For this review, take the finished solid that the model builds, in its own axes (mm). A direction names the side the tool comes from. Give positions to 0.01 mm unless a question says otherwise; leave off trailing zeros. Order: outer loops, then holes, each group sorted by start corner. A loop starts at its lowest first (then second) coordinate and runs counter-clockwise, first axis right, second up. Notation, with made-up numbers: (25, -34) - (56, -34) arc R20 cw to (56, -12) - close; hole circle Ø1 at (34, 16.25). An arc over 180 degrees is marked (long way). Use a Markdown table: item, result. Add a question column.
1) We need section A-A on x = 4.75. Write out the cut boundary in (y, z).
2) Machinability: for faces 4 (the face through (-7.25, 0.65, 0.5)), 5 (the face through (-1, 7, 0)), 6 (the face through (-4.61, -4.987, 0.501)), 7 (the face through (-6.28, 4.25, 0.5)), which of the approach directions +Z, -Z, +X, -X, +Y, -Y give a long, thin tool a straight path to every point of the face, cutting with its end or side? Answer none if there is none.
3) Wall thickness on L1, parallel to Z at x = 2.25, y = -4.25; L2, parallel to Z at x = 5, y = -6.5; L3, parallel to Y at x = 6.75, z = 0.4: over which ranges is each line inside the solid? List them lowest first.
4) We need section B-B on z = -1. Write out the cut boundary in (x, y) (3 decimals), then the cut area to 3 significant figures.
5) Clearance check with flat-ended pins moving along their axes: P1, Ø1, axis at y = 4.5, z = -1.5, coming from the -X side; P2, Ø0.5, axis at x = 0, z = 0.5, coming from the -Y side; P3, Ø7, axis at x = -0.5, y = -3.5, coming from the +Z side; P4, Ø0.5, axis at y = 0.5, z = 0.5, coming from the +X side. State where each tip first meets the part, or that it passes through.
6) Mouldability with a two-part tool opening along X and no side actions: class faces 1 (the face through (-0.1, -8.666, 0.5)), 2 (the face through (-2.85, -7.1, 0.5)), 3 (the face through (0, 1, 0.762)) as released by +X, released by -X, zero draft, split by the parting line, or undercut.
```python
from build123d import *

# Parameters (mm, degrees)
F2_DEPTH  = 1.016
F0_R      = 9.525
F3_DEPTH  = 1.778
F5_DEPTH  = 0.73658
F8_DEPTH  = 0.19799
F10_DEPTH = 0.254
F12_DEPTH = 0.254
F14_DEPTH = 0.254
F16_DEPTH = 0.13808
F18_DEPTH = 0.254


with BuildPart() as f2:
    # F1 (on Top) → F2 (new body)
    with BuildSketch(Plane.XY):
        Polygon((-5.2096517757, 4.8718452454), (-7.3895002715, 3.6098279525), (-6.5481550992, 2.3594415264), (-6.86526423, 2.3594415264), (-7.3371550568, 1.5301066978), (-6.8923411891, 1.2770079775), (-7.6189576648, 0), (-7.6189576648, -0.3674388281), (-7.1600424126, -2.2795863915), (-6.7776124924, -3.1974171288), (-5.4391096346, -4.4211917557), (-3.7564195227, -5.5684801191), (-1.9207580481, -8.6661595851), (1.8270511646, -8.6661595851), (4.0068994276, -5.4537514225), (5.4983743466, -4.6506496146), (7.0280926302, -2.9297166038), (7.639979478, -1.7441851087), (7.639979478, -0.7116254419), (7.639979478, 0.3974201391), (7.639979478, 1.0475503514), (7.639979478, 1.6976804473), (6.4162053168, 2.4625393562), (7.6782228425, 3.6098279525), (5.6895888411, 4.5659020543), (4.427571781, 5.7131904177), (3.471497912, 6.1338627711), (1.6740793362, 7.0134503767), (0, 6.36332063), (-1.5000854619, 6.9752074778), (-3.2975040376, 6.17210567), (-4.3683070689, 5.5219754577), align=None)
    extrude(amount=F2_DEPTH)

    # F0 (on Top) → F3 (join)
    with BuildSketch(Plane.XY):
        Circle(F0_R)
    extrude(amount=-F3_DEPTH)

    # F7 (on face) → F8 (cut)
    with BuildSketch(Plane.XY.offset(1.016)):
        Polygon((-1.3463342329, 6.4942925237), (-2.822693903, 5.8646216057), (-2.6447118726, 5.755500868), (-1.3636830263, 6.2029086985), (0, 5.3883814253), (1.3446520315, 6.2008285895), (2.729951404, 5.569380708), (2.881785389, 5.6656086817), (1.3232411584, 6.5193735063), (0, 5.8390707709), align=None)
    extrude(amount=-F8_DEPTH, mode=Mode.SUBTRACT)

    # F9 (on face) → F10 (cut)
    with BuildSketch(Plane.XY.offset(1.016)):
        Polygon((-3.0135090929, -4.5730909333), (-2.8008187655, -4.5092836954), (-3.4176206682, -2.6801475324), (-4.5236102305, -2.1271528676), (-5.7784831151, -0.2554782841), (-5.1404121332, 0.4251306527), (-5.4594473913, 1.2333536288), (-5.246757064, 2.679647645), (-5.5232541636, 2.679647645), (-6.3314777799, 0.5314758164), (-6.3314777799, -1.0211633053), (-4.0769609623, -3.9137513377), (-3.545235144, -3.9137513377), align=None)
        Polygon((5.5232541636, 2.679647645), (5.246757064, 2.679647645), (5.4594473913, 1.2333536288), (5.1404121332, 0.4251306527), (5.7784831151, -0.2554782841), (4.5236102305, -2.1271528676), (3.4176206682, -2.6801475324), (2.8008187655, -4.5092836954), (3.0135090929, -4.5730909333), (3.545235144, -3.9137513377), (4.0769609623, -3.9137513377), (6.3314777799, -1.0211633053), (6.3314777799, 0.5314758164), align=None)
    extrude(amount=-F10_DEPTH, mode=Mode.SUBTRACT)

    # F11 (on face) → F12 (cut)
    with BuildSketch(Plane.XY.offset(1.016)):
        Polygon((0, 0), (-3.1052604318, -0.9244027315), (-1.7141137505, -7.7665727586), (0, -7.0284130052), (1.820534002, -7.7665727586), (3.1832898967, -0.938598183), align=None)
    extrude(amount=-F12_DEPTH, mode=Mode.SUBTRACT)

    # F13 (on face) → F14 (cut)
    with BuildSketch(Plane.XY.offset(1.016)):
        Polygon((-1.822640141, 2.3322773777), (0, 0.2859818342), (1.7637592973, 2.2436233703), (1.6359017026, 2.3588181173), (0.7133174804, 1.6945287352), (-0.5281137419, 1.6945287352), (-1.7337343888, 2.4704232346), align=None)
        Polygon((-2.1157131996, 3.043391509), (-1.4591871295, 3.7715386134), (-1.9366606139, 4.3086963706), (-3.9181755856, 4.4996854849), (-2.5812499225, 3.043391509), align=None)
        Polygon((1.4591871295, 3.7715386134), (2.1157131996, 3.043391509), (2.5812499225, 3.043391509), (3.9181755856, 4.4996854849), (1.9366606139, 4.3086963706), align=None)
    extrude(amount=-F14_DEPTH, mode=Mode.SUBTRACT)

    # F15 (on face) → F16 (join)
    with BuildSketch(Plane.XY.offset(0.762)):
        with BuildLine():
            Line((2.5812499225, 3.043391509), (2.7644233944, 3.2429197483))
            ThreePointArc((2.7644233944, 3.2429197483), (2.3504007339, 3.7546674576), (1.9342565257, 3.2446434588))
            Line((1.9342565257, 3.2446434588), (2.1157131996, 3.043391509))
            Line((2.1157131996, 3.043391509), (2.5812499225, 3.043391509))
        make_face()
        with BuildLine():
            Line((-2.7644233944, 3.2429197483), (-2.5812499225, 3.043391509))
            Line((-2.5812499225, 3.043391509), (-2.1157131996, 3.043391509))
            Line((-2.1157131996, 3.043391509), (-1.9342565257, 3.2446434588))
            ThreePointArc((-1.9342565257, 3.2446434588), (-2.3504007339, 3.7546674576), (-2.7644233944, 3.2429197483))
        make_face()
    extrude(amount=F16_DEPTH)

    # F17 (on face) → F18 (cut)
    with BuildSketch(Plane.XY.offset(0.762)):
        Polygon((-1.6513522714, -0.8654528065), (-2.665983513, -1.2116211001), (-2.0300412055, -3.8737652845), (-1.8184679793, -3.8854728919), align=None)
        Polygon((-1.5797313536, -7.1800402366), (-0.9351419867, -6.9413036108), (-1.4483418965, -4.579841237), (-1.6871627886, -4.5897462405), align=None)
        Polygon((1.5797313536, -7.1800402366), (1.6871627886, -4.5897462405), (1.4483418965, -4.579841237), (0.9351419867, -6.9413036108), align=None)
        Polygon((1.6513522714, -0.8654528065), (1.8184679793, -3.8854728919), (2.0300412055, -3.8737652845), (2.665983513, -1.2116211001), align=None)
        Polygon((0.1592475164, -0.9012632072), (-0.1592475164, -0.9012632072), (-1.2335629435, -0.9012632072), (-1.4842365636, -1.9158945652), (-1.2574365828, -1.9158945652), (-0.803836796, -1.283242018), (-0.5292895366, -1.6413471894), (-0.1250742725, -1.3314488641), (0.1250742725, -1.3314488641), (0.5292895366, -1.6413471894), (0.803836796, -1.283242018), (1.2574365828, -1.9158945652), (1.4842365636, -1.9158945652), (1.2335629435, -0.9012632072), align=None)
        Polygon((-0.6731920876, -6.11623656), (-0.6731920876, -6.9274515845), (-0.1211152558, -6.9274515845), (0.1211152558, -6.9274515845), (0.6731920876, -6.9274515845), (0.6731920876, -6.11623656), (0.5548899644, -6.11623656), (0.2788515121, -6.6401464865), (0, -6.2683396973), (-0.2788515121, -6.6401464865), (-0.5548899644, -6.11623656), align=None)
    extrude(amount=-F18_DEPTH, mode=Mode.SUBTRACT)


with BuildPart() as f5:
    # F4 (on face) → F5 (new body)
    with BuildSketch(Plane.XY.offset(1.016)):
        Polygon((17.713438698, 4.5463088655), (15.3496832919, 3.1778191726), (16.2620100905, 1.8219416059), (15.9181474671, 1.8219416059), (15.4064447065, 0.9226384258), (15.8887861108, 0.6481865685), (15.1008673055, -0.7365585255), (15.1008673055, -1.1349970032), (15.5984997833, -3.2084663974), (16.013194104, -4.2037316056), (17.4646222066, -5.5307522199), (19.2892755512, -6.7748336671), (21.2798059676, -10.1338545338), (25.3438059676, -10.1338545338), (27.7075611212, -6.6504256738), (29.324867053, -5.7795687113), (30.9836428208, -3.9134460356), (31.647152623, -2.6278950049), (31.647152623, -1.508221551), (31.647152623, -0.3056093086), (31.647152623, 0.3993703296), (31.647152623, 1.1043498415), (30.3201325137, 1.933737473), (31.688622459, 3.1778191726), (29.5322137084, 4.2145542169), (28.163724268, 5.458635664), (27.1269894762, 5.9147988108), (25.1779283908, 6.8685944355), (23.3626122858, 6.1636153022), (21.7359693669, 6.8271251044), (19.7869082815, 5.9562681419), (18.6257649916, 5.2512885037), align=None)
        Polygon((18.439305509, 1.7165624937), (18.4358818544, 1.7216506446), (19.9132289832, 2.5769567026), (20.4834329167, 3.0175689765), (21.2091474729, 3.4581812504), (22.4273106513, 4.0024668519), (23.4439624756, 3.5877732256), (23.4679646927, 3.5970945015), (25.3034550697, 4.8505836166), (25.7937528554, 3.4337042665), (25.7966982196, 3.4322629184), (26.4446574645, 3.1471609517), (27.2999633647, 2.3696100472), (28.6477188339, 1.7216506446), (28.6426317994, 1.7170260681), (28.6477188339, 1.7145803783), (27.7970213842, 0.9412191032), (28.6218001864, 0.4257323126), (28.6218001864, 0.4186620463), (28.6218001864, -0.5960899286), (28.6218001864, -0.6644358361), (28.6218001864, -1.0367022025), (28.6218001864, -1.1050481099), (28.6218001864, -1.7883348539), (28.6218001864, -1.8566807614), (28.6218001864, -1.9069207164), (28.6218001864, -1.9139909827), (28.20710656, -2.7174603769), (27.1703717051, -3.8837870492), (26.1595554977, -4.4280726508), (24.6822085267, -6.6052156882), (22.1422085267, -6.6052156882), (20.8981270165, -4.5058276465), (19.7577186761, -3.7282767421), (18.850576112, -2.8988888581), (18.5913921616, -2.276848103), (18.2803718629, -0.9809297316), (18.2803718629, -0.9738594653), (18.2803718629, -0.7319056831), (18.2803718629, -0.7248354168), (18.7697820642, 0.1352892187), (18.4713577386, 0.3050924115), (18.4743967906, 0.3104334598), (18.4713577386, 0.3121626778), (18.7911719639, 0.8742271654), (19.0013287467, 0.8742271654), (18.4358818544, 1.7145803783), align=None, mode=Mode.SUBTRACT)
    extrude(amount=F5_DEPTH)


solid = f2.part
```
Checked values:
| question | item | result |
|---|---|---|
| 1 | outline | (-8.26, -1.78) - (8.26, -1.78) - (8.26, 0) - (5.42, 0) - (5.42, 1.02) - (-1.79, 1.02) - (-1.79, 0.76) - (-3.05, 0.76) - (-3.05, 1.02) - (-5.05, 1.02) - (-5.05, 0) - (-8.26, 0) - close |
| 2 | face 4 | +Z, -X |
| 2 | face 5 | +Z |
| 2 | face 6 | +Z, -X, -Y |
| 2 | face 7 | +Z, -X, +Y |
| 3 | L1 | -1.78 to 0.76 |
| 3 | L2 | -1.78 to 0 |
| 3 | L3 | -3.24 to 2.25, 2.77 to 4.06 |
| 4 | outline | circle Ø19.05 at (0, 0) |
| 4 | area | 285 mm² |
| 5 | P1 | x = -8.64 |
| 5 | P2 | y = -8.67 |
| 5 | P3 | z = 1.02 |
| 5 | P4 | x = 7.64 |
| 6 | face 1 | zero draft |
| 6 | face 2 | released by -X |
| 6 | face 3 | undercut |
